Source: CAD feature listing. Evaluate the final solid. Frame: model axes, mm. Give positions to 0.01 mm unless a question says otherwise; leave off trailing zeros. Order: outer loops, then holes, each group sorted by start corner. A loop starts at its lowest first (then second) coordinate and runs counter-clockwise, first axis right, second up. Notation, with made-up numbers: M 11.5,72.5 L 31.5,72.5 A22 ccw 31.5,103.5 Z; hole C -24.75,74.5 d5. An arc over 180 degrees is marked long. Answer as a JSON object with one key per item and string values. Group by question number.
1. Section query C-C (z = 2.85). Count the separate pieces of the cut face and the enclosed holes in it, plus the area to 3 significant figures.
2. Section query D-D (x = -66). Output: boundary loops of the cut face in (y, z), plus the area to 3 significant figures.
3. Material intervals for L1, parallel to Y at x = -4.5, z = 0.25; L2, parallel to Y at x = -5.5, z = 3.75; L3, parallel to Y at x = 41, z = 1.45, sorted ascending. Write a range as [from, to].
4. Section query B-B (x = 44.5). Output: boundary loops of the cut face in (y, z), plus the area to 3 significant figures.
5. Section query A-A (x = -8.5). Output: boundary loops of the cut face in (y, z).
6. Pin query (flat end, axial travel): P1, Ø2, axis at x = -73, z = 1.5, coming from the +Y side; P2, Ø1, axis at y = -18.5, z = 2, coming from the -X side; P3, Ø2, axis at x = 30, z = 2, coming from the +Y side. Return the tip coordinate at first contact, or that it passes through.
from build123d import *

# Parameters (mm, degrees)
SKETCH_1_R      = 1.5
SKETCH_1_R_2    = 3
SKETCH_1_R_3    = 1.25
SKETCH_1_R_4    = 2
SKETCH_1_W      = 4.3
SKETCH_1_H      = 8.3
EXTRUDE_1_DEPTH = 4
FILLET_1_R      = 1.3
FILLET_2_R      = 2


with BuildPart() as part:
    # 草图1 → 凸台-拉伸1 (new body)
    with BuildSketch(Plane.XY):
        with BuildLine():
            Line((32.115707856, 27.15), (32.115707856, 22.85))
            Line((32.115707856, 22.85), (27.815707856, 22.85))
            Line((27.815707856, 22.85), (27.815707856, 27.15))
            Line((27.815707856, 27.15), (-29.075, 27.15))
            Line((-29.075, 27.15), (-38.998995168, 22.002009663))
            ThreePointArc((-38.998995168, 22.002009663), (-52.370174504, 17.472835843), (-60.236366221, 5.75))
            Line((-60.236366221, 5.75), (-80.958287312, 5.75))
            Line((-80.958287312, 5.75), (-80.958287312, -5.75))
            Line((-80.958287312, -5.75), (-60.236366221, -5.75))
            ThreePointArc((-60.236366221, -5.75), (-52.370174504, -17.472835843), (-38.998995168, -22.002009663))
            Line((-38.998995168, -22.002009663), (-29.075, -27.15))
            Line((-29.075, -27.15), (27.815707856, -27.15))
            Line((27.815707856, -27.15), (27.815707856, -22.85))
            Line((27.815707856, -22.85), (32.115707856, -22.85))
            Line((32.115707856, -22.85), (32.115707856, -27.15))
            Line((32.115707856, -27.15), (36.001004832, -27.15))
            Line((36.001004832, -27.15), (52.659242152, -27.15))
            Line((52.659242152, -27.15), (52.659242152, -14.15))
            Line((52.659242152, -14.15), (36.001004832, -14.15))
            Line((36.001004832, -14.15), (36.001004832, 27.15))
            Line((36.001004832, 27.15), (32.115707856, 27.15))
        make_face()
        with Locations((30.001004832, 13.5)):
            Circle(SKETCH_1_R, mode=Mode.SUBTRACT)
        with Locations(Location((30.001004832, -13.5, 0), (0, 0, 180))):
            Circle(SKETCH_1_R, mode=Mode.SUBTRACT)
        with Locations((-38.998995168, 0)):
            Circle(SKETCH_1_R_2, mode=Mode.SUBTRACT)
        with Locations((-38.998995168, -11.5)):
            Circle(SKETCH_1_R_3, mode=Mode.SUBTRACT)
        with Locations((-48.958287312, -5.75)):
            Circle(SKETCH_1_R_3, mode=Mode.SUBTRACT)
        with Locations((-48.958287312, 5.75)):
            Circle(SKETCH_1_R_3, mode=Mode.SUBTRACT)
        with Locations((-38.998995168, 11.5)):
            Circle(SKETCH_1_R_3, mode=Mode.SUBTRACT)
        with Locations((-29.039703025, 5.75)):
            Circle(SKETCH_1_R_3, mode=Mode.SUBTRACT)
        with Locations((-29.039703025, -5.75)):
            Circle(SKETCH_1_R_3, mode=Mode.SUBTRACT)
        with Locations((-4.075, -22.15)):
            Circle(SKETCH_1_R_4, mode=Mode.SUBTRACT)
        with Locations((-4.075, 22.15)):
            Circle(SKETCH_1_R_4, mode=Mode.SUBTRACT)
        with Locations((-76.958287312, 0)):
            Circle(SKETCH_1_R_4, mode=Mode.SUBTRACT)
        with Locations((30.001004832, 0)):
            Rectangle(SKETCH_1_W, SKETCH_1_H, mode=Mode.SUBTRACT)
        Polygon((-21.039703025, -1.433615613), (-2.627787708, -13.528909152), (22.001004832, -7.277030256), (22.001004832, 7.277030256), (-2.627787708, 13.528909152), (-21.039703025, 1.433615613), align=None, mode=Mode.SUBTRACT)
    extrude(amount=EXTRUDE_1_DEPTH)

    # 圆角1
    fillet_1_edges = [part.edges().sort_by_distance(p)[0] for p in [
        (-29.075, -27.15, 2),
        (-60.236366221, -5.75, 2),
        (-80.958287312, -5.75, 2),
        (-80.958287312, 5.75, 2),
        (-60.236366221, 5.75, 2),
        (-29.075, 27.15, 2),
        (52.659242152, -14.15, 2),
        (52.659242152, -27.15, 2),
    ]]
    fillet(fillet_1_edges, radius=FILLET_1_R)

    # 圆角2
    fillet_2_edges = [part.edges().sort_by_distance(p)[0] for p in [
        (-21.039703025, 1.433615613, 2),
        (-21.039703025, -1.433615613, 2),
        (-2.627787708, -13.528909152, 2),
        (22.001004832, -7.277030256, 2),
        (22.001004832, 7.277030256, 2),
        (-2.627787708, 13.528909152, 2),
    ]]
    fillet(fillet_2_edges, radius=FILLET_2_R)


solid = part.part
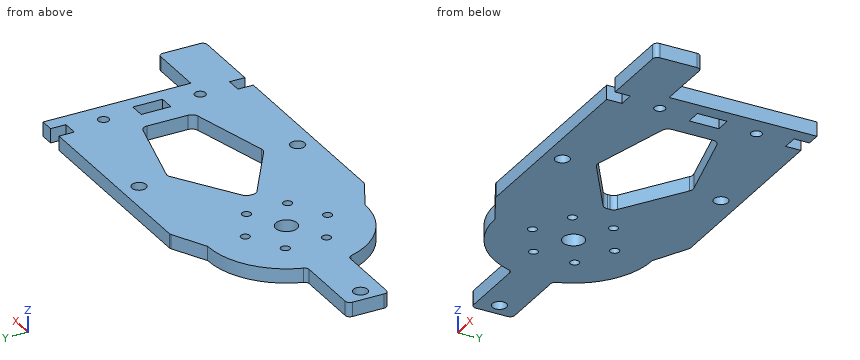
Answer sheet:
{
 "1": {"separate pieces": "1", "enclosed holes": "14", "area": "4,260 mm^2"},
 "2": {"outline": "M -5.75,0 L 5.75,0 L 5.75,4 L -5.75,4 Z", "area": "46.0 mm^2"},
 "3": {"L1": "[-27.15, -24.1], [-20.2, -12.3], [12.3, 20.2], [24.1, 27.15]", "L2": "[-27.15, -23.55], [-20.75, -11.64], [11.64, 20.75], [23.55, 27.15]", "L3": "[-27.15, -14.15]"},
 "4": {"outline": "M -27.15,0 L -14.15,0 L -14.15,4 L -27.15,4 Z", "area": "52.0 mm^2"},
 "5": {"outline": "M -27.15,0 L -9.67,0 L -9.67,4 L -27.15,4 Z; M 9.67,0 L 27.15,0 L 27.15,4 L 9.67,4 Z"},
 "6": {"P1": "y = 5.75", "P2": "x = -51.65", "P3": "y = 22.85"}
}
